Job drawing, mm, ordinate dimensions from the low corner. One solid piece. Coordinates: 2 decimals unless noted, no trailing zeros. Loops run counter-clockwise (first coordinate to the right, second up) from the corner with the lowest first, then second, coordinate; pieces in that order, holes last. Notation, with made-up numbers: (-35, -35) - (-12, -35) arc R29 cw to (-12, -12) - close; hole circle Ø8 at (-34.75, 8). An arc over 180 degrees is marked (long way). Use a Markdown table: item, result. Add a question column.
1. Drop flat-ended pins along their axis: pin 1 (0.9 mm diameter, centred on x = 1, z = 1.5, fed in from -Y); pin 2 (1.5 mm diameter, centred on y = 51, z = 2, fed in from -X); pin 3 (12 mm diameter, centred on x = 36.5, y = 19.4, fed in from -Z); pin 4 (1.5 mm diameter, centred on x = 71.5, z = 2, fed in from +Y). Give the stop position or say it passes through.
2. Band-saw the part on C-C, the plane y = 13. Give the cut face in (x, z), plus the area to 3 significant figures.
3. Wall check: probe 1 along Y at (x, z) = (37, 0.9); probe 2 along X at (y, z) = (45, 2.3); probe 3 along Y at (x, z) = (7.5, 2.75). Give the ranges that are in metal, low to high. Write a range as [from, to].
4. Band-saw the part on A-A, the plane x = 36.5. Give the cut face in (y, z), plus the area to 3 significant figures.
5. Band-saw the part on D-D, the plane x = 6. Give the cut face in (y, z).
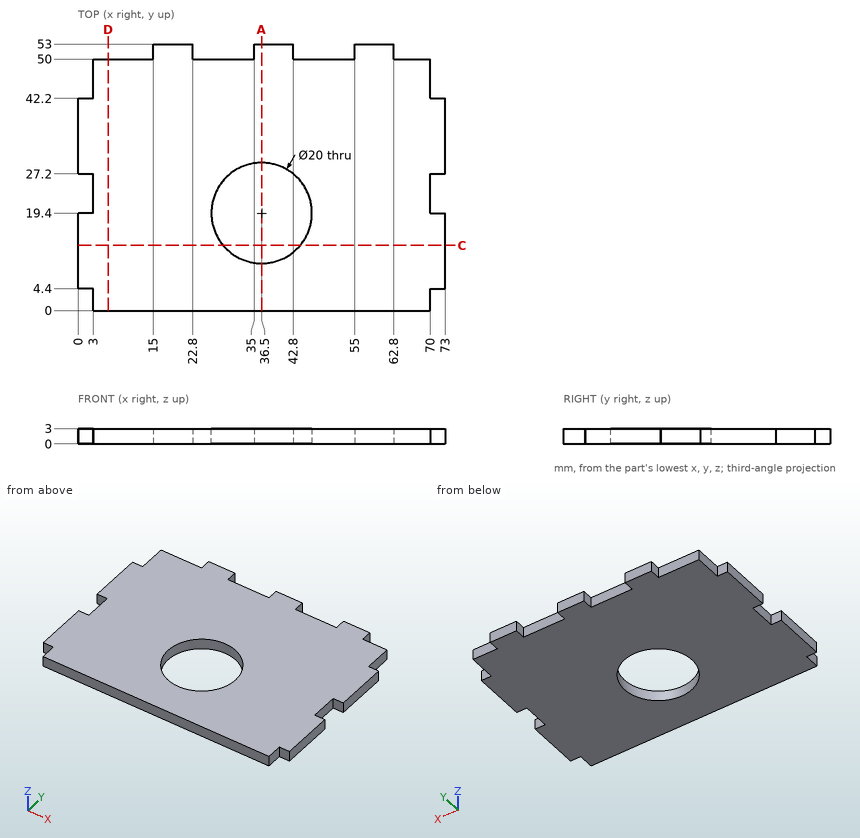
Geometry check:
| question | item | result |
|---|---|---|
| 1 | pin 1 | stops at y = 4.4 |
| 1 | pin 2 | stops at x = 15 |
| 1 | pin 3 | passes through |
| 1 | pin 4 | stops at y = 42.2 |
| 2 | outline | (0, 0) - (28.82, 0) - (28.82, 3) - (0, 3) - close; (44.18, 0) - (73, 0) - (73, 3) - (44.18, 3) - close |
| 2 | area | 173 mm^2 |
| 3 | probe 1 | y = [0, 9.41], [29.39, 53] |
| 3 | probe 2 | x = [3, 70] |
| 3 | probe 3 | y = [0, 50] |
| 4 | outline | (0, 0) - (9.4, 0) - (9.4, 3) - (0, 3) - close; (29.4, 0) - (53, 0) - (53, 3) - (29.4, 3) - close |
| 4 | area | 99.0 mm^2 |
| 5 | outline | (0, 0) - (50, 0) - (50, 3) - (0, 3) - close |
